Read the model definition and answer for the solid it produces. Units are mm, in the model's axes. Face numbers are marked on the shaded views. A direction names the side the tool comes from. Coordinates: 2 decimals unless noted, no trailing zeros. Write each loop counter-clockwise with the first axis right and the second up, starting at its lowest first coordinate (ties: lowest second). Pieces come first, ordered by that corner, then holes. Notation, with made-up numbers: M -35.5,3.5 L -31.5,3.5 A19 cw -31.5,40.5 Z; hole C -8,-15 d8. An arc over 180 degrees is marked long. Write item = value, one per line.
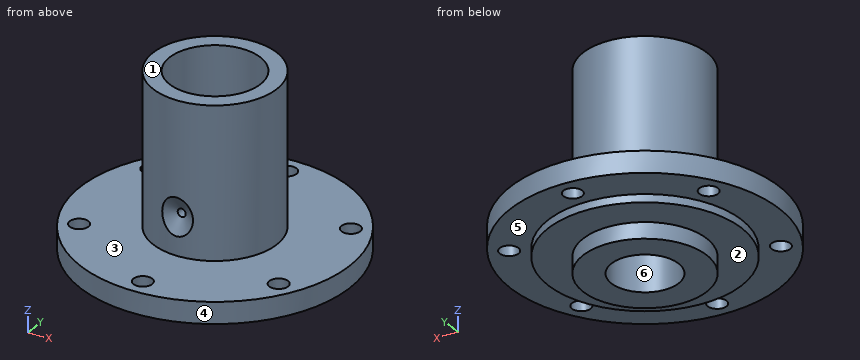
Autodesk Inventor part; units mm, degrees
ref_plane "Work Plane1" through (0, -23, 8.5) normal (0, 1, 0) x (-1, 0, 0)
ref_plane "YZ Plane" through (0, 0, 0) normal (1, 0, 0) x (0, 1, 0)
ref_plane "XY Plane" through (0, 0, 0) normal (0, 0, 1) x (1, 0, 0)
sketch "Sketch1" plane through (0, 0, 0) normal (0, 1, 0) x (-1, 0, 0)
  line L0 (0, -36.5) -> (-23, -36.5)
  line L1 (-23, -36.5) -> (-23, 36.5)
  line L2 (-23, 36.5) -> (0, 36.5)
  line L3 (0, 36.5) -> (0, -36.5)
  line L4 (-23, -30.5) -> (-36, -30.5)
  line L5 (-36, -30.5) -> (-36, -27.5)
  line L6 (-36, -27.5) -> (-50, -27.5)
  line L7 (-50, -27.5) -> (-50, -19.5)
  line L8 (-50, -19.5) -> (-23, -19.5)
  point P0 (0, 0)
  point P1 (0, 0)
  dimension "d0" = 73
  dimension "d1" = 46
  dimension "d2" = 72
  dimension "d3" = 100
  dimension "d5" = 3
  dimension "d6" = 8
  dimension "d41" = 9
revolve "Revolution1" add sketch "Sketch1" angle 360 about axis through (0, 0, 36.5) along (0, 0, -1)
sketch "Sketch2" plane through (0, 0, -36.5) normal (0, 0, -1) x (-1, 0, 0)
  point P0 (0, 0)
hole "Hole1" at (0, 0, -36.5) direction (0, 0, 1) diameter 25 end through all
sketch "Sketch3" plane through (0, 0, 36.5) normal (0, 0, 1) x (1, 0, 0)
  point P0 (0, 0)
hole "Hole2" at (0, 0, 36.5) direction (0, 0, -1) diameter 33.835 depth 23
ref_plane "Work Plane1" through (0, -23, 8.5) normal (0, 1, 0) x (-1, 0, 0)
sketch "Sketch4" plane through (0, -23, 8.5) normal (0, 1, 0) x (-1, 0, 0)
  line L0 (23, 28) -> (-23, 28) construction
  point P0 (0, -8.5)
  point P1 (0, -14)
  dimension "d22" = 42
hole "Hole3" at (0, -23, -5.5) direction (0, 1, 0) diameter 3 end up to surface countersink diameter 14 countersink angle 120
sketch "Sketch5" plane through (0, 0, -19.5) normal (0, 0, 1) x (1, 0, 0)
  circle A0 centre (0, 0) radius 12.5
  circle A1 centre (0, 0) radius 43 construction
  point P0 (0, 0)
  point P1 (0, -43)
  dimension "d30" = 86
hole "Hole4" at (0, -43, -19.5) direction (0, 0, -1) diameter 7 end through all
pattern_circular "Circular Pattern1" count 6 over 360 about axis through (0, 0, -10) along (0, 0, 1) of "Hole4"
properties material "Aluminum 6061"
Item 1: Consider line 1 along X through (y, z) = (0, 19); line 2 along X through (y, z) = (0, -16). Determine where each line is inside the solid, lowest interval first. Write a range as from..to.
Worked answers:
line_1 = -23..-16.92, 16.92..23
line_2 = -23..-12.5, 12.5..23
Item 2: Find section D-D (x = -31.5). Determine the outline of the cut face in (y, z), and give its area (3 significant figures).
Worked answers:
outline = M -38.83,-27.5 L -17.43,-27.5 L -17.43,-30.5 L 17.43,-30.5 L 17.43,-27.5 L 38.83,-27.5 L 38.83,-19.5 L -38.83,-19.5 Z
area = 726 mm²
Item 3: For a pull along X with two mould halves and no side action, classify the marked faces 4, 5 and 6 as released by +X, released by -X, zero draft, split by the parting line, or undercut.
Worked answers:
face_4 = split by the parting line
face_5 = zero draft
face_6 = undercut
Item 4: Find section B-B (y = 0). Determine the outline of the cut face in (x, z).
Worked answers:
outline = M -50,-27.5 L -36,-27.5 L -36,-30.5 L -23,-30.5 L -23,-36.5 L -12.5,-36.5 L -12.5,13.5 L -16.92,13.5 L -16.92,36.5 L -23,36.5 L -23,-19.5 L -50,-19.5 Z; M 12.5,-36.5 L 23,-36.5 L 23,-30.5 L 36,-30.5 L 36,-27.5 L 50,-27.5 L 50,-19.5 L 23,-19.5 L 23,36.5 L 16.92,36.5 L 16.92,13.5 L 12.5,13.5 Z
Item 5: Flat-ended cylindrical pins translate along their axes: pin 1 (8 mm diameter, centred on x = -37.24, y = 21.5, fed in from +Z); pin 2 (9 mm diameter, centred on x = 0, y = -43, fed in from -Z); pin 3 (6 mm diameter, centred on x = 2.5, z = 18, fed in from +Y). Find the tip coordinate at first contact, or state that the pin passes through.
Worked answers:
pin_1 = -19.5
pin_2 = -27.5
pin_3 = 23
Item 6: Which of the six approach directions +Z, -Z, +X, -X, +Y, -Y give full straight-line access (tool end or side, diameter ignored) to the marked faces 1, 2 and 3?
Worked answers:
face_1 = +Z, +X, -X, +Y, -Y
face_2 = -Z
face_3 = +Z
Item 7: Find section C-C (z = 30.5). Determine the outline of the cut face in (x, y) (1 decimal).
Worked answers:
outline = C 0,0 d46; hole C 0,0 d33.8
Item 8: Find section A-A (y = -21.5). Determine the outline of the cut face in (x, z), and give its area (3 significant figures).
Worked answers:
outline = M -45.14,-27.5 L -40.74,-27.5 L -40.74,-19.5 L -45.14,-19.5 Z; M -33.74,-27.5 L -28.87,-27.5 L -28.87,-30.5 L -8.17,-30.5 L -8.17,-36.5 L 8.17,-36.5 L 8.17,-30.5 L 28.87,-30.5 L 28.87,-27.5 L 33.74,-27.5 L 33.74,-19.5 L 8.17,-19.5 L 8.17,36.5 L -8.17,36.5 L -8.17,-19.5 L -33.74,-19.5 Z; M 40.74,-27.5 L 45.14,-27.5 L 45.14,-19.5 L 40.74,-19.5 Z; hole C 0,-5.5 d8.8
area = 1,740 mm²
